from build123d import *

# Parameters (mm, degrees)
ESBO_O1_R                  = 1.9
RESSALTO_EXTRUS_O1_DEPTH   = 3
RESSALTO_EXTRUS_O3_DEPTH   = 28
CORTE_EXTRUS_O_FINA4_START = -3.000000318
CORTE_EXTRUS_O_FINA4_DEPTH = 3.000000318
PADR_OCIRCULAR1_COUNT      = 2
ESBO_O5_R                  = 0.5
CORTE_EXTRUS_O5_DEPTH      = 2


# Read off the part's stored shape, not the designer's step: Corte-Extrusão-Fina4
with BuildPart() as part:
    # Esboço1 → Ressalto-extrusão1 (new body)
    with BuildSketch(Plane.XY):
        Circle(ESBO_O1_R)
    extrude(amount=RESSALTO_EXTRUS_O1_DEPTH)

    # Esboço4 → Ressalto-extrusão3 (add)
    with BuildSketch(Plane(origin=(0, 0, 0), x_dir=(0, 0, -1), z_dir=(1, 0, 0))):
        with BuildLine():
            Line((0, 2.966582109), (-0.302284292, 2.966582109))
            add(Edge.make_bspline(
                [(-0.302284292, 2.966582109), (-0.48011033, 0.989335618), (-1.388364091, -2.104701367), (-3, -3.303217097)],
                knots=[0, 0, 0, 0, 1, 1, 1, 1], degree=3))
            Line((-3, -3.303217097), (-2.572366731, -3.303217097))
            add(Edge.make_bspline(
                [(0, 2.966582109), (-0.177826038, 0.989335618), (-1.013540392, -2.259955739), (-2.572366731, -3.303217097)],
                knots=[0, 0, 0, 0, 1, 1, 1, 1], degree=3))
        make_face()
    ressalto_extrus_o3 = extrude(amount=RESSALTO_EXTRUS_O3_DEPTH)

    # Corte-Extrusão-Fina4 outline → Corte-Extrusão-Fina4 (cut)
    with BuildSketch(Plane.XY.offset(3).offset(CORTE_EXTRUS_O_FINA4_START)):
        with BuildLine():
            add(Edge.make_bspline(
                [(15.965244027, 2.966582109), (22.160101016, 2.966582102), (27.105451106, 2.406382612), (27.65, 1.185252223)],
                knots=[0.449610583, 0.449610583, 0.449610583, 0.449610583, 1, 1, 1, 1], degree=3))
            add(Edge.make_bspline(
                [(27.65, 1.185252223), (27.943589962, 1.15875623), (28.093651275, -1.845186793), (27.691880485, -1.884412653)],
                knots=[0, 0, 0, 0, 1, 1, 1, 1], degree=3))
            add(Edge.make_bspline(
                [(27.691880485, -1.884412653), (25.053075141, -2.604086837), (21.639173149, -3.168169457), (17.53715106, -3.303217097), (15.849087583, -3.303217097)],
                knots=[0, 0, 0, 0, 0.243203402, 0.407668544, 0.407668544, 0.407668544, 0.407668544], degree=3))
            Line((15.849087583, -3.303217097), (28, -3.303217097))
            Line((28, -3.303217097), (28, 2.966582109))
            Line((28, 2.966582109), (15.965244027, 2.966582109))
        make_face()
        with BuildLine():
            add(Edge.make_bspline(
                [(0, 1.9), (5.010325131, 2.59275087), (10.904693859, 2.966582115), (15.965244027, 2.966582109)],
                knots=[0, 0, 0, 0, 0.449610583, 0.449610583, 0.449610583, 0.449610583], degree=3))
            Line((15.965244027, 2.966582109), (0, 2.966582109))
            Line((0, 2.966582109), (0, 1.9))
        make_face()
        with BuildLine():
            Line((0, -3.303217097), (15.849087583, -3.303217097))
            add(Edge.make_bspline(
                [(15.849087583, -3.303217097), (9.769421811, -3.303217097), (3.259233415, -2.59651639), (0, -1.9)],
                knots=[0.407668544, 0.407668544, 0.407668544, 0.407668544, 1, 1, 1, 1], degree=3))
            Line((0, -1.9), (0, -3.303217097))
        make_face()
    corte_extrus_o_fina4 = extrude(amount=CORTE_EXTRUS_O_FINA4_DEPTH, mode=Mode.SUBTRACT)

    # PadrãoCircular1: Ressalto-extrusão3, Corte-Extrusão-Fina4 ×2 about axis
    padr_ocircular1_axis = Axis((0, 0, 3), (0, 0, -1))
    add([ressalto_extrus_o3.rotate(padr_ocircular1_axis, i * 360 / PADR_OCIRCULAR1_COUNT) for i in range(1, PADR_OCIRCULAR1_COUNT)])
    add([corte_extrus_o_fina4.rotate(padr_ocircular1_axis, i * 360 / PADR_OCIRCULAR1_COUNT) for i in range(1, PADR_OCIRCULAR1_COUNT)], mode=Mode.SUBTRACT)

    # Esboço5 → Corte-extrusão5 (cut)
    with BuildSketch(Plane.XY.offset(3)):
        Circle(ESBO_O5_R)
    extrude(amount=-CORTE_EXTRUS_O5_DEPTH, mode=Mode.SUBTRACT)


solid = part.part
Read the model definition and answer for the solid it produces. Units are mm, in the model's axes. A direction names the side the tool comes from. Coordinates: 2 decimals unless noted, no trailing zeros. Answer in a Markdown table with one row per item.
Q1. Given P1, Ø2, axis at x = -19, y = -1, coming from the +Z side; P2, Ø0.5, axis at x = 0, y = 0, coming from the +Z side; P3, Ø2, axis at x = 7, y = -0.5, coming from the -Z side, each flat-ended and moving along its own axis, determine where each tip first touches the part or whether it passes through.
Here are the results:
| item | result |
|---|---|
| P1 | stops at z = 0.95 |
| P2 | stops at z = 1 |
| P3 | stops at z = 0.45 |
Q2. For faces 1 (the flat face through (0, 0, 0)), 2 (the cylindrical face through (-0.108, -0.488, 2.014)), 3 (the cylindrical face through (-0.412, -1.855, 1.479)), determine the directions among +Z, -Z, +X, -X, +Y, -Y from which every point of the face is accessible in a straight line to the end or side of a thin tool.
Here are the results:
| item | result |
|---|---|
| face 1 | -Z, +X, -X, +Y, -Y |
| face 2 | +Z |
| face 3 | none |
Q3. The mould has two halves that part along X. Classify faces 4 (the flat face through (1, 0, 3)), 5 (the flat face through (0, 0, 1)): pulls with the +X half, pulls with the -X half, needs draft (parallel to the pull), parting line crosses it, or undercut.
Here are the results:
| item | result |
|---|---|
| face 4 | needs draft |
| face 5 | undercut |
Q4. Straight lines are drawn through the part: line 1 along Y through (x, z) = (0, 1.7); line 2 along Z through (x, y) = (-2, 1); line 3 along Z through (x, y) = (-15, 2.25). For each, find the intervals that lie inside material, in ascending order. Write a range as [from, to].
Here are the results:
| item | result |
|---|---|
| line 1 | y = [-1.9, -0.5], [0.5, 1.9] |
| line 2 | z = [0.95, 1.34] |
| line 3 | z = [1.59, 2.03] |
